from build123d import *

# Parameters (mm, degrees)
EXTRUDE_1_DEPTH     = 10
SKETCH_2_R          = 6
CUT_EXTRUDE_1_DEPTH = 11
SKETCH_3_R          = 14
SKETCH_3_R_2        = 1.7
CUT_EXTRUDE_2_DEPTH = 11


with BuildPart() as part:
    # Эскиз1 → Бобышка-Вытянуть1 (new body)
    with BuildSketch(Plane(origin=(0, 0, 0), x_dir=(1, 0, 0), z_dir=(0, 1, 0))):
        Polygon((42, 0.149999792), (89.999875, 0.149999792), (89.999875, 45), (0, 45), (0, 0), (0, -42), (42, -42), align=None)
    extrude(amount=EXTRUDE_1_DEPTH)

    # Эскиз2 → Вырез-Вытянуть1 (cut, through all)
    with BuildSketch(Plane(origin=(0, 10, 0), x_dir=(1, 0, 0), z_dir=(0, 1, 0))):
        with Locations((67.5, 22.5)):
            Circle(SKETCH_2_R)
        with Locations((22.5, 22.5)):
            Circle(SKETCH_2_R)
    extrude(amount=-CUT_EXTRUDE_1_DEPTH, mode=Mode.SUBTRACT)

    # Эскиз3 → Вырез-Вытянуть2 (cut, through all)
    with BuildSketch(Plane(origin=(0, 10, 0), x_dir=(1, 0, 0), z_dir=(0, 1, 0))):
        with Locations((20.959394321, -21.15)):
            Circle(SKETCH_3_R)
        with Locations((33.333762992, -33.524368671)):
            Circle(SKETCH_3_R_2)
        with Locations((8.585025651, -33.524368671)):
            Circle(SKETCH_3_R_2)
        with Locations((8.585025651, -8.775631329)):
            Circle(SKETCH_3_R_2)
        with Locations((33.333762992, -8.775631329)):
            Circle(SKETCH_3_R_2)
    extrude(amount=-CUT_EXTRUDE_2_DEPTH, mode=Mode.SUBTRACT)


solid = part.part
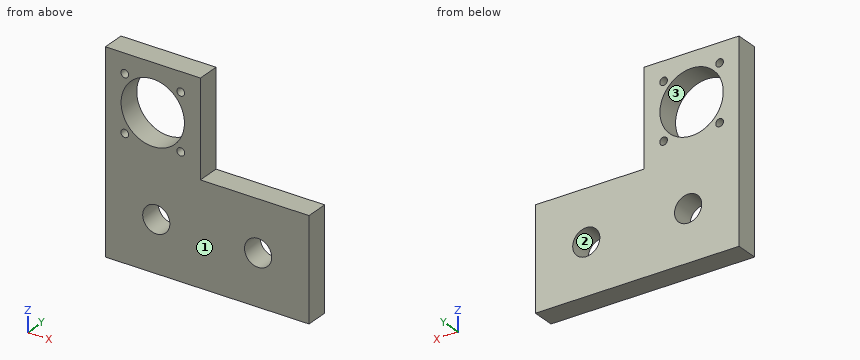
Source: CAD feature listing. Evaluate the final solid. Frame: model axes, mm. Face numbers are marked on the shaded views. Round coordinates to 2 decimals unless told otherwise and drop trailing zeros. Loops run counter-clockwise (first coordinate to the right, second up) from the corner with the lowest first, then second, coordinate; pieces in that order, holes last. Notation, with made-up numbers: (75, 86) - (96, 86) arc R24 cw to (96, 120) - close; hole circle Ø8 at (50, -35). An arc over 180 degrees is marked (long way). Write item = value, one per line. Start each with the question number.
Item 1: Section query D-D on x = 22.5. Output: boundary loops of the cut face in (y, z).
Item 2: Mould query, pull axis Z, two halves, no side actions, for the marked faces 1, 2 and 3. Classes: released by +Z, released by -Z, zero draft, split by the parting line, or undercut.
Item 3: Section query C-C on z = 21.15. Output: boundary loops of the cut face in (x, y).
Item 4: Material intervals for line 1 (X direction, y = 4, z = -22.5); line 2 (X direction, y = 7.5, z = 32.5); line 3 (Z direction, x = 67.5, y = 5.75), sorted ascending.
Item 5: Section query B-B on x = 67.5. Output: boundary loops of the cut face in (y, z), plus the area to 4 significant figures.
Item 6: Section query A-A on z = -22.5. Output: boundary loops of the cut face in (x, y), plus the area to 3 significant figures.
Item 7: First-contact query: pin 1 Ø5 at (x, y) = (71.5, 5.5) entering from +Z. Flat tip, straight axial feed; report the tip coordinate or a pass-through.
Results list:
q1.outline = (0, -45) - (10, -45) - (10, -28.5) - (0, -28.5) - close; (0, -16.5) - (10, -16.5) - (10, 7.24) - (0, 7.24) - close; (0, 35.06) - (10, 35.06) - (10, 42) - (0, 42) - close
q2.face_1 = zero draft
q2.face_2 = undercut
q2.face_3 = undercut
q3.outline = (0, 0) - (6.96, 0) - (6.96, 10) - (0, 10) - close; (34.96, 0) - (42, 0) - (42, 10) - (34.96, 10) - close
q4.line_1 = 0 to 16.5, 28.5 to 61.5, 73.5 to 90
q4.line_2 = 0 to 7.23, 9.94 to 12.76, 29.16 to 31.98, 34.69 to 42
q4.line_3 = -45 to -28.5, -16.5 to -0.15
q5.outline = (0, -45) - (10, -45) - (10, -28.5) - (0, -28.5) - close; (0, -16.5) - (10, -16.5) - (10, -0.15) - (0, -0.15) - close
q5.area = 328.5 mm²
q6.outline = (0, 0) - (16.5, 0) - (16.5, 10) - (0, 10) - close; (28.5, 0) - (61.5, 0) - (61.5, 10) - (28.5, 10) - close; (73.5, 0) - (90, 0) - (90, 10) - (73.5, 10) - close
q6.area = 660 mm²
q7.pin_1 = -0.15
